Design review of the part built by this model. Coordinates are the model's own, in mm. Give positions to 0.01 mm unless a question says otherwise; leave off trailing zeros. Write each loop counter-clockwise with the first axis right and the second up, starting at its lowest first coordinate (ties: lowest second). Pieces come first, ordered by that corner, then holes. Notation, with made-up numbers: (28.25, -21.75) -> (57.25, -21.75) arc R20 ccw to (57.25, -16.75) -> close; hole circle Ø3 at (-29, -31). An arc over 180 degrees is marked (long way). Answer as a JSON object with one key per item and string values.
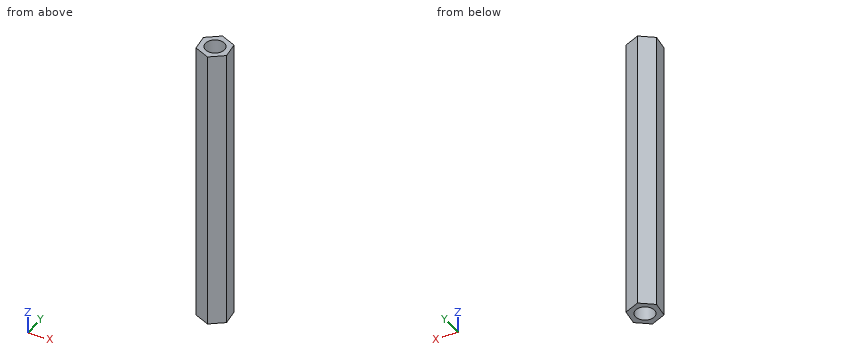
```python
from build123d import *

# Parameters (mm, degrees)
EXTRUDE_1_DEPTH          = 60
SKETCH_2_R               = 2
CUT_EXTRUDE_1_DEPTH      = 1
CUT_EXTRUDE_1_DEPTH_BACK = 61


with BuildPart() as part:
    # 草图1 → 凸台-拉伸1 (new body)
    with BuildSketch(Plane.XY):
        Polygon((2.759819518, 2.093656186), (-0.433249685, 3.436901906), (-3.193069203, 1.34324572), (-2.759819518, -2.093656186), (0.433249685, -3.436901906), (3.193069203, -1.34324572), align=None)
    extrude(amount=EXTRUDE_1_DEPTH)

    # 草图2 → 切除-拉伸1 (cut, two sides)
    with BuildSketch(Plane.XY.offset(60)) as cut_extrude_1_sk:
        Circle(SKETCH_2_R)
    extrude(amount=CUT_EXTRUDE_1_DEPTH, mode=Mode.SUBTRACT)
    extrude(cut_extrude_1_sk.sketch, amount=-CUT_EXTRUDE_1_DEPTH_BACK, mode=Mode.SUBTRACT)


solid = part.part
```
(1) We need section B-B, the plane y = 0. State the section outline as (x, z) points, then the cut area to 3 significant figures.
Here are the results:
{"outline": "(-3.02, 0) -> (-2, 0) -> (-2, 60) -> (-3.02, 60) -> close; (2, 0) -> (3.02, 0) -> (3.02, 60) -> (2, 60) -> close", "area": "123 mm²"}
(2) For line 1 along X through (y, z) = (0.25, 27); line 2 along Y through (x, z) = (0.75, 8); line 3 along Y through (x, z) = (0, 36), list the stretches that pass through material, from the lowest coordinate up.
Here are the results:
{"line 1": "x = -3.06 to -1.98, 1.98 to 2.99", "line 2": "y = -3.2 to -1.85, 1.85 to 2.94", "line 3": "y = -3.25 to -2, 2 to 3.25"}
(3) Clearance check with flat-ended pins moving along their axes: pin 1 (1.5 mm diameter, centred on y = 0.5, z = 43.5, fed in from -X); pin 2 (2.5 mm diameter, centred on x = 0, y = 0, fed in from -Z); pin 3 (1 mm diameter, centred on y = 2.5, z = 13.5, fed in from -X); pin 4 (2 mm diameter, centred on y = -2, z = 19, fed in from -X). State where each tip first meets the part, or that it passes through.
Here are the results:
{"pin 1": "stops at x = -3.18", "pin 2": "passes through", "pin 3": "stops at x = -2.33", "pin 4": "stops at x = -2.9"}
(4) We need section A-A, the plane z = 27. State the section outline as (x, y) points, then the cut area to 3 significant figures.
Here are the results:
{"outline": "(-3.19, 1.34) -> (-2.76, -2.09) -> (0.43, -3.44) -> (3.19, -1.34) -> (2.76, 2.09) -> (-0.43, 3.44) -> close; hole circle Ø4 at (0, 0)", "area": "18.6 mm²"}
